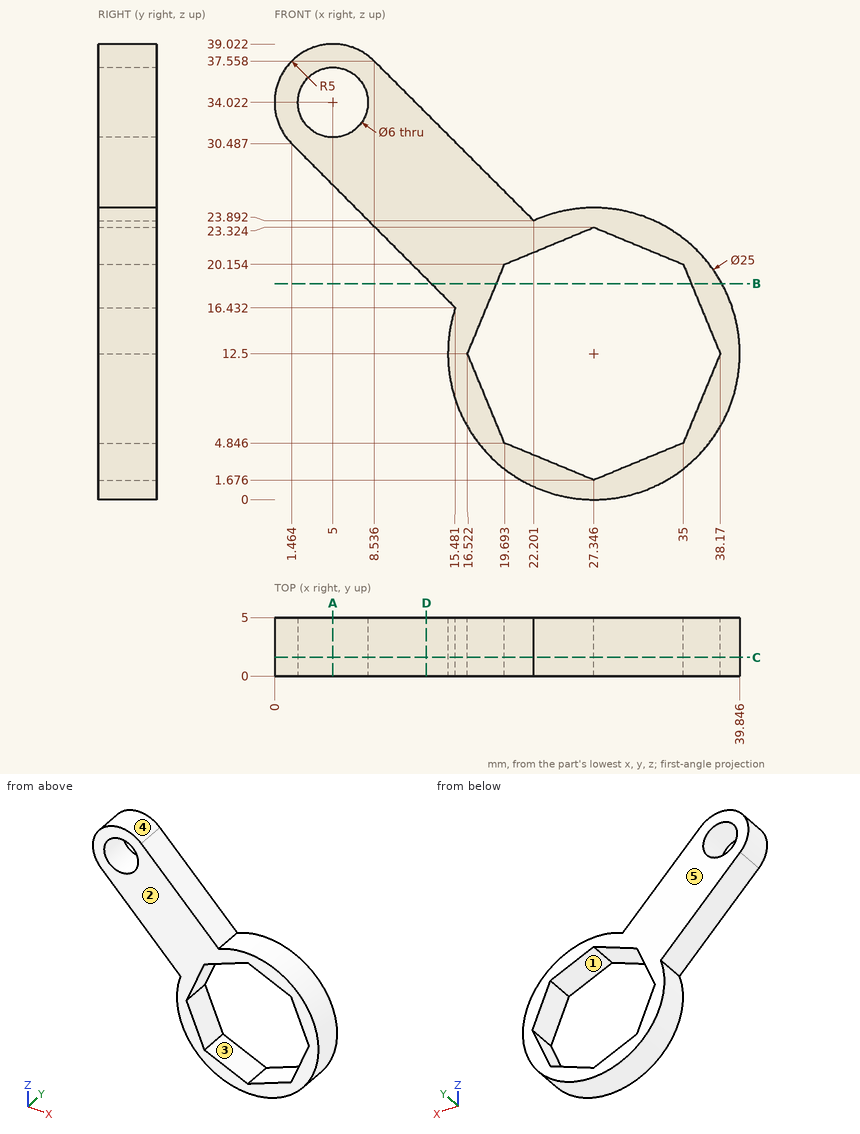
The drawing under review shows one solid part. Ordinate dimensions are in mm from its lowest x, y, z. A direction names the side the tool comes from. Round coordinates to 2 decimals unless told otherwise and drop trailing zeros. Write each loop counter-clockwise with the first axis right and the second up, starting at its lowest first coordinate (ties: lowest second). Pieces come first, ordered by that corner, then holes. Notation, with made-up numbers: (34, -1.75) - (74, -1.75) arc R20 ccw to (74, 10.25) - close; hole circle Ø5 at (22.25, 67.5). An arc over 180 degrees is marked (long way). Use one line per item in the form item = value.
Q1. Consider section D-D (x = 13). State the section outline as (y, z) points.
Answer key:
outline = (0, 18.92) - (5, 18.92) - (5, 33.09) - (0, 33.09) - close
Q2. Consider section B-B (z = 18.5). State the section outline as (x, y) points (1 decimal).
Answer key:
outline = (13.4, 0) - (19, 0) - (19, 5) - (13.4, 5) - close; (35.7, 0) - (38.3, 0) - (38.3, 5) - (35.7, 5) - close
Q3. Consider section C-C (y = 1.6). State the section outline as (x, z) points (1 decimal).
Answer key:
outline = (1.5, 30.5) - (15.5, 16.4) arc R12.5 ccw (long way) to (22.2, 23.9) - (8.5, 37.6) arc R5 ccw to start; hole circle Ø6 at (5, 34); hole (16.5, 12.5) - (19.7, 4.8) - (27.3, 1.7) - (35, 4.8) - (38.2, 12.5) - (35, 20.2) - (27.3, 23.3) - (19.7, 20.2) - close
Q4. For line 1 (Z direction, x = 36, y = 0.4) (1 decimal); line 2 (Z direction, x = 4.5, y = 3.9) (1 decimal); line 3 (X direction, y = 3.65, z = 2) (1 decimal), list the stretches that pass through material, from the lowest coordinate up. Write a range as [from, to].
Answer key:
line_1 = [3.5, 7.3], [17.7, 21.5]
line_2 = [27.4, 31.1], [37, 39]
line_3 = [20.6, 26.6], [28.1, 34.1]
Q5. Tool access review of the marked faces 1 and 2: name each direction out of +Z, -Z, +X, -X, +Y, -Y from which nothing blocks a thin tool from reaching the whole face with its end or side.
Answer key:
face_1 = +Y, -Y
face_2 = +Z, -Z, +X, -X, -Y
Q6. Consider section A-A (x = 5). State the section outline as (y, z) points, and give its area (3 significant figures).
Answer key:
outline = (0, 26.94) - (5, 26.94) - (5, 31.02) - (0, 31.02) - close; (0, 37.02) - (5, 37.02) - (5, 39.02) - (0, 39.02) - close
area = 30.4 mm2
Q7. Insertion check: pin 1 Ø1 at (x, y) = (13, 4) entering from +Z (1 decimal); pin 2 Ø1 at (x, z) = (16.5, 30.5) entering from -Y. Each pin has a flat end and moves straight along its axis. Give the tip position at first contact, or say it passes through.
Answer key:
pin_1 = 33.6
pin_2 = through
Q8. Draft analysis for pull direction X (two halves, no side actions). For the marked faces 3, 4 and 5, state which applies: +X half, -X half, draft (parallel to the pull), parting line (faces both ways), or undercut.
Answer key:
face_3 = undercut
face_4 = parting line
face_5 = draft
